Here's the drawing with two shaded views (mm, measured from the low corner). I have some questions. A direction names the side the tool comes from. Give positions to 0.01 mm unless a question says otherwise; leave off trailing zeros. Loops run counter-clockwise (first coordinate to the right, second up) from the corner with the lowest first, then second, coordinate; pieces in that order, holes last. Notation, with made-up numbers: (37.5, 19) - (86.5, 19) arc R18 ccw to (86.5, 30) - close; hole circle Ø10 at (85, -1.5). An arc over 180 degrees is marked (long way). Write each question's results on one line, items separated by ' | '. Start each with the question number.
1) I want a section at C-C, the plane z = 58. Write out the boundary of the cut face in (x, y).
2) I want a section at B-B, the plane y = 6.5. Write out the boundary of the cut face in (x, z), and give its area (3 significant figures).
3) I'm going to push flat-ended pins straight in: pin 1 (2 mm diameter, centred on x = 8.5, z = 61, fed in from -Y); pin 2 (1 mm diameter, centred on x = 3, z = 32, fed in from -Y); pin 3 (5 mm diameter, centred on x = 8, z = 28.5, fed in from -Y). Where does each tip first touch, or does it pass through?
4) If I drill on probe 1 along Z at (x, y) = (11.25, 12.75); probe 2 along Y at (x, z) = (4, 27); probe 3 along X at (y, z) = (1.75, 16), over which ranges is the centre line in solid material (lowest first)? Write a range as [from, to].
5) On a 3-axis mill with a long thin cutter (end or side, diameter ignored), from which of +Z, -Z, +X, -X, +Y, -Y can I reach the whole of each face in a straight line? I mean the marked faces 1, 2 and 3. Say none if no direction works.
6) I want a section at A-A, the plane x = 9.75. Write out the boundary of the cut face in (y, z).
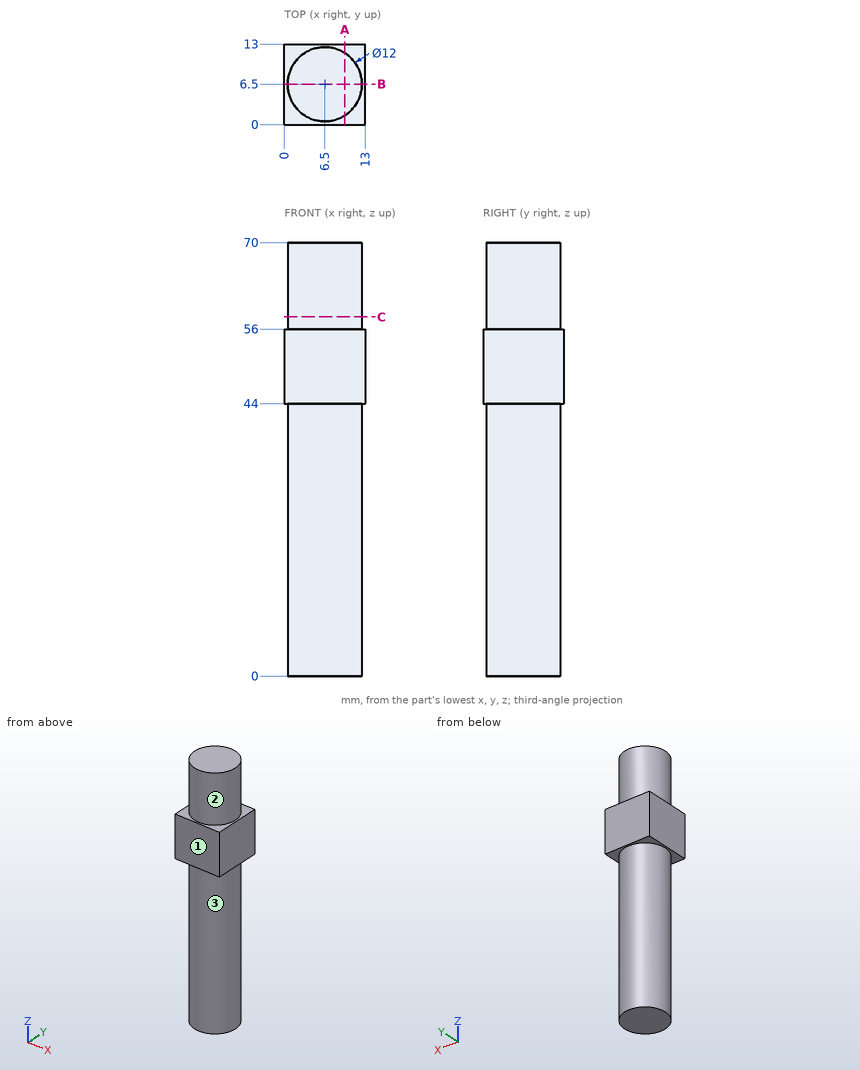
Answers:
1) outline: circle Ø12 at (6.5, 6.5)
2) outline: (0, 44) - (0.5, 44) - (0.5, 0) - (12.5, 0) - (12.5, 44) - (13, 44) - (13, 56) - (12.5, 56) - (12.5, 70) - (0.5, 70) - (0.5, 56) - (0, 56) - close | area: 852 mm2
3) pin 1: stops at y = 0.58 | pin 2: stops at y = 1.3 | pin 3: stops at y = 0.5
4) probe 1: z = [44, 56] | probe 2: y = [1.05, 11.95] | probe 3: x = [2.83, 10.17]
5) face 1: +Z, -Z, +X, -X, -Y | face 2: +Z | face 3: -Z
6) outline: (0, 44) - (1.46, 44) - (1.46, 0) - (11.54, 0) - (11.54, 44) - (13, 44) - (13, 56) - (11.54, 56) - (11.54, 70) - (1.46, 70) - (1.46, 56) - (0, 56) - close
